Geometry check sheet. Reference: the model listing, model coordinates, mm. Coordinates: 2 decimals unless noted, no trailing zeros. Order: outer loops, then holes, each group sorted by start corner. A loop starts at its lowest first (then second) coordinate and runs counter-clockwise, first axis right, second up. Notation, with made-up numbers: (36.25, 16.5) - (57.25, 16.5) arc R15 cw to (57.25, 37.5) - close; hole circle Ø8 at (21, 22.5). An arc over 180 degrees is marked (long way). Return JSON: item names as keys, results as strings. Group by question number.
Item 1: Section check B-B on y = 0. Enter the section's corners in (x, z).
Item 2: Section check C-C on x = -49. Enter the section's corners in (y, z).
Item 3: Gauge pin test, flat ends, axial feed: pin 1 (1 mm diameter, centred on x = 25.5, z = 1, fed in from -Y); pin 2 (1 mm diameter, centred on x = -33.5, z = 2, fed in from +Y); pin 3 (5 mm diameter, centred on x = 0, y = -61.5, fed in from +Z). Record the tip position at first contact, or that the pin passes through.
Item 4: Section check A-A on x = 0. Enter the section's corners in (y, z).
Item 5: Draft check along X on faces 1 (the cylindrical face through (42.837, 40.558, 1.479)), 2 (the flat face through (15, 1, 3)), 3 (the cylindrical face through (-9.373, 71.387, 1.479)), 4 (the cylindrical face through (-0.59, 4.46, 1.48)). Enter one of: pulls with the +X half, pulls with the -X half, needs draft (parallel to the pull), parting line crosses it, or undercut.
Item 6: Scan lines: probe 1 along Y at (x, z) = (0, 0.7); probe 2 along X at (y, z) = (-41, 2.85); probe 3 along Y at (x, z) = (-41.5, 0.75). Record each from-to range of solid material in increasing order.
Item 7: Section check D-D on y = 61.5. Enter the section's corners in (x, z), then the cut area to 3 significant figures.
from build123d import *

# Parameters (mm, degrees)
F0_R     = 72
F0_R_2   = 3
F0_R_3   = 25.35
F0_R_4   = 4.5
F1_DEPTH = 3


with BuildPart() as f1:
    # F0 (on Top) → F1 (new body)
    with BuildSketch(Plane.XY):
        Circle(F0_R)
        with Locations((-43.487067, -43.487067)):
            Circle(F0_R_2, mode=Mode.SUBTRACT)
        with Locations((0, -61.5)):
            Circle(F0_R_2, mode=Mode.SUBTRACT)
        with Locations((-40.65, 0)):
            Circle(F0_R_3, mode=Mode.SUBTRACT)
        Circle(F0_R_4, mode=Mode.SUBTRACT)
        with Locations((0, 61.5)):
            Circle(F0_R_2, mode=Mode.SUBTRACT)
        with Locations((43.487067, 43.487067)):
            Circle(F0_R_2, mode=Mode.SUBTRACT)
    extrude(amount=F1_DEPTH)


solid = f1.part
Computed:
{
 "1": {"outline": "(-72, 0) - (-66, 0) - (-66, 3) - (-72, 3) - close; (-15.3, 0) - (-4.5, 0) - (-4.5, 3) - (-15.3, 3) - close; (4.5, 0) - (72, 0) - (72, 3) - (4.5, 3) - close"},
 "2": {"outline": "(-52.75, 0) - (-23.94, 0) - (-23.94, 3) - (-52.75, 3) - close; (23.94, 0) - (52.75, 0) - (52.75, 3) - (23.94, 3) - close"},
 "3": {"pin 1": "stops at y = -67.52", "pin 2": "stops at y = 63.99", "pin 3": "passes through"},
 "4": {"outline": "(-72, 0) - (-64.5, 0) - (-64.5, 3) - (-72, 3) - close; (-58.5, 0) - (-4.5, 0) - (-4.5, 3) - (-58.5, 3) - close; (4.5, 0) - (58.5, 0) - (58.5, 3) - (4.5, 3) - close; (64.5, 0) - (72, 0) - (72, 3) - (64.5, 3) - close"},
 "5": {"face 1": "undercut", "face 2": "needs draft", "face 3": "parting line crosses it", "face 4": "undercut"},
 "6": {"probe 1": "y = -72 to -64.5, -58.5 to -4.5, 4.5 to 58.5, 64.5 to 72", "probe 2": "x = -59.19 to -45.16, -41.81 to 59.19", "probe 3": "y = -58.84 to -45.73, -41.24 to -25.34, 25.34 to 58.84"},
 "7": {"outline": "(-37.44, 0) - (-3, 0) - (-3, 3) - (-37.44, 3) - close; (3, 0) - (37.44, 0) - (37.44, 3) - (3, 3) - close", "area": "207 mm²"}
}
